CAD build for the part. Positions are in the model's coordinates, mm. Face numbers are marked on the shaded views. Coordinates: 2 decimals unless noted, no trailing zeros. Loops run counter-clockwise (first coordinate to the right, second up) from the corner with the lowest first, then second, coordinate; pieces in that order, holes last. Notation, with made-up numbers: (79.25, -33) -> (107.25, -33) arc R11 cw to (107.25, -14) -> close; hole circle Ø3 at (-15, 64.25). An arc over 180 degrees is marked (long way). Return JSON: item names as keys, results as strings. Group by question number.
(1) Saw through at C-C on y = 15. Write the cut outline in (x, z).
(2) Saw through at B-B on z = 3.5. Write the cut outline in (x, y), then the cut area to 3 significant figures.
(3) Mould opens along X. For the marked faces 1 and 2 say: pulls with the +X half, pulls with the -X half, needs draft (parallel to the pull), parting line crosses it, or undercut.
(4) Flat gauge pins, fed straight in: pin 1 Ø4.5 at (x, y) = (-30.1, 30.1) entering from +Z; pin 2 Ø5 at (x, z) = (-20, 5) entering from +Y; pin 3 Ø1.5 at (y, z) = (26.5, 7.5) entering from +X; pin 4 Ø6 at (x, y) = (3.5, -27) entering from +Z. Where does each tip first touch, or does it go through?
(5) Saw through at A-A on z = 8. Write the cut outline in (x, y).
(6) Probe L1, parallel to Y at x = -30.1, z = 1.05; L2, parallel to Y at x = -30.1, z = 7.05; L3, parallel to Y at x = 30.1, z = 4.75. List the from-to ranges inside material, lowest first.
```python
from build123d import *

# Parameters (mm, degrees)
SKETCH1_W                                  = 80.2
SKETCH1_H                                  = 80.2
BOSS_EXTRUDE1_DEPTH                        = 4.5
M5_CLEARANCE_HOLE1_D                       = 5.5
FILLET2_R                                  = 10
SKETCH3_R                                  = 4.5
BOSS_EXTRUDE2_DEPTH                        = 6
CUT_EXTRUDE1_REACH                         = 59.026
SKETCH5_R                                  = 2.75
MIRROR2_AT_THE_SECOND_PLANE_COPY_1_SKETC_R = 4.5
MIRROR2_AT_THE_SECOND_PLANE_COPY_1_DEPTH   = 6
MIRROR2_AT_THE_SECOND_PLANE_COPY_2_REACH   = 59.026
MIRROR2_AT_THE_SECOND_PLANE_COPY_2_SKETC_R = 2.75
FILLET4_R                                  = 1


with BuildPart() as part:
    # Sketch1 → Boss-Extrude1 (new body)
    with BuildSketch(Plane.XY):
        Rectangle(SKETCH1_W, SKETCH1_H)
    extrude(amount=BOSS_EXTRUDE1_DEPTH)

    # M5 Clearance Hole1 (through all)
    with Locations(Plane(origin=(-30.1, -30.1, 0), x_dir=(-1, 0, 0), z_dir=(0, 0, -1))):
        with Locations((0, 0), (-60.2, 60.2), (0, 60.2), (-60.2, 0)):
            Hole(M5_CLEARANCE_HOLE1_D / 2)

    # Fillet2
    fillet2_edges = [part.edges().sort_by_distance(p)[0] for p in [
        (40.1, -40.1, 2.25),
        (-40.1, -40.1, 2.25),
        (-40.1, 40.1, 2.25),
        (40.1, 40.1, 2.25),
    ]]
    fillet(fillet2_edges, radius=FILLET2_R)

    # Sketch3 → Boss-Extrude2 (add)
    with BuildSketch(Plane.XY.offset(4.5)):
        with Locations(Location((-30.1, 30.1, 0), (0, 0, 180))):
            Circle(SKETCH3_R)
    boss_extrude2 = extrude(amount=BOSS_EXTRUDE2_DEPTH)

    # Sketch5 → Cut-Extrude1 (cut, up to next)
    with BuildSketch(Plane(origin=(0, 0, 4.5), x_dir=(-1, 0, 0), z_dir=(0, 0, -1)), mode=Mode.PRIVATE) as cut_extrude1_sk1:
        with Locations((30.1, 30.1)):
            Circle(SKETCH5_R)
    cut_extrude1_tool1 = extrude(cut_extrude1_sk1.sketch, amount=-CUT_EXTRUDE1_REACH, mode=Mode.PRIVATE) & part.part
    cut_extrude1 = cut_extrude1_tool1.solids().sort_by_distance((-30.1, 30.1, 4.5))[0]
    add(cut_extrude1, mode=Mode.SUBTRACT)

    # Mirror2: Boss-Extrude2, Cut-Extrude1 across plane
    add(boss_extrude2.mirror(Plane.ZX))
    add(cut_extrude1.mirror(Plane.ZX), mode=Mode.SUBTRACT)

    # Mirror2 at the second plane: Boss-Extrude2, Cut-Extrude1 across plane
    add(boss_extrude2.mirror(Plane(origin=(0, 0, 0), x_dir=(0, 0, 1), z_dir=(1, 0, 0))))
    add(cut_extrude1.mirror(Plane(origin=(0, 0, 0), x_dir=(0, 0, 1), z_dir=(1, 0, 0))), mode=Mode.SUBTRACT)

    # Mirror2 at the second plane copy 1 sketc → Mirror2 at the second plane copy 1 (add)
    with BuildSketch(Plane(origin=(0, 0, 4.5), x_dir=(-1, 0, 0), z_dir=(0, 0, 1))):
        with Locations(Location((-30.1, 30.1, 0), (0, 0, 180))):
            Circle(MIRROR2_AT_THE_SECOND_PLANE_COPY_1_SKETC_R)
    extrude(amount=MIRROR2_AT_THE_SECOND_PLANE_COPY_1_DEPTH)

    # Mirror2 at the second plane copy 2 sketc → Mirror2 at the second plane copy 2 (cut, up to next)
    with BuildSketch(Plane(origin=(0, 0, 4.5), x_dir=(1, 0, 0), z_dir=(0, 0, -1)), mode=Mode.PRIVATE) as mirror2_at_the_second_plane_copy_2_sk1:
        with Locations((30.1, 30.1)):
            Circle(MIRROR2_AT_THE_SECOND_PLANE_COPY_2_SKETC_R)
    mirror2_at_the_second_plane_copy_2_tool1 = extrude(mirror2_at_the_second_plane_copy_2_sk1.sketch, amount=-MIRROR2_AT_THE_SECOND_PLANE_COPY_2_REACH, mode=Mode.PRIVATE) & part.part
    add(mirror2_at_the_second_plane_copy_2_tool1.solids().sort_by_distance((30.1, -30.1, 4.5))[0], mode=Mode.SUBTRACT)

    # Fillet4
    fillet4_edges = [part.edges().sort_by_distance(p)[0] for p in [
        (-25.6, 30.1, 4.5),
        (25.6, 30.1, 4.5),
        (-25.6, -30.1, 4.5),
        (25.6, -30.1, 4.5),
    ]]
    fillet(fillet4_edges, radius=FILLET4_R)


solid = part.part
```
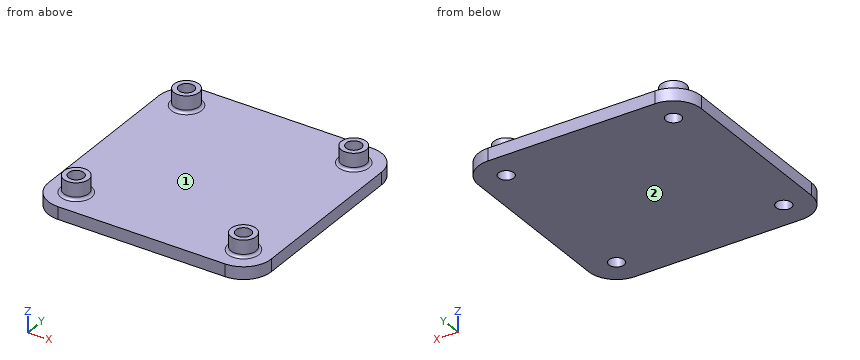
Geometry results:
{
 "1": {"outline": "(-40.1, 0) -> (40.1, 0) -> (40.1, 4.5) -> (-40.1, 4.5) -> close"},
 "2": {"outline": "(-40.1, -30.1) arc R10 ccw to (-30.1, -40.1) -> (30.1, -40.1) arc R10 ccw to (40.1, -30.1) -> (40.1, 30.1) arc R10 ccw to (30.1, 40.1) -> (-30.1, 40.1) arc R10 ccw to (-40.1, 30.1) -> close; hole circle Ø5.5 at (-30.1, -30.1); hole circle Ø5.5 at (-30.1, 30.1); hole circle Ø5.5 at (30.1, -30.1); hole circle Ø5.5 at (30.1, 30.1)", "area": "6,250 mm²"},
 "3": {"face 1": "undercut", "face 2": "needs draft"},
 "4": {"pin 1": "through", "pin 2": "y = 40.1", "pin 3": "x = 33.58", "pin 4": "z = 4.5"},
 "5": {"outline": "circle Ø9 at (-30.1, -30.1); circle Ø9 at (-30.1, 30.1); circle Ø9 at (30.1, -30.1); circle Ø9 at (30.1, 30.1); hole circle Ø5.5 at (-30.1, -30.1); hole circle Ø5.5 at (-30.1, 30.1); hole circle Ø5.5 at (30.1, -30.1); hole circle Ø5.5 at (30.1, 30.1)"},
 "6": {"L1": "-40.1 to -32.85, -27.35 to 27.35, 32.85 to 40.1", "L2": "-34.6 to -32.85, -27.35 to -25.6, 25.6 to 27.35, 32.85 to 34.6", "L3": "-34.94 to -32.85, -27.35 to -25.26, 25.26 to 27.35, 32.85 to 34.94"}
}
